The listing builds one solid part. Answer for the finished solid, in the listing's coordinates (mm). Face numbers are marked on the shaded views. A direction names the side the tool comes from. Give positions to 0.01 mm unless a question says otherwise; leave off trailing zeros. Loops run counter-clockwise (first coordinate to the right, second up) from the corner with the lowest first, then second, coordinate; pieces in that order, holes last. Notation, with made-up numbers: (51.25, 42.5) -> (90.25, 42.5) arc R19 ccw to (90.25, 48.5) -> close; hole circle Ø8 at (-37, 2). An arc over 180 degrees is marked (long way). One line per question, with ' | ' between items. Start each with the question number.
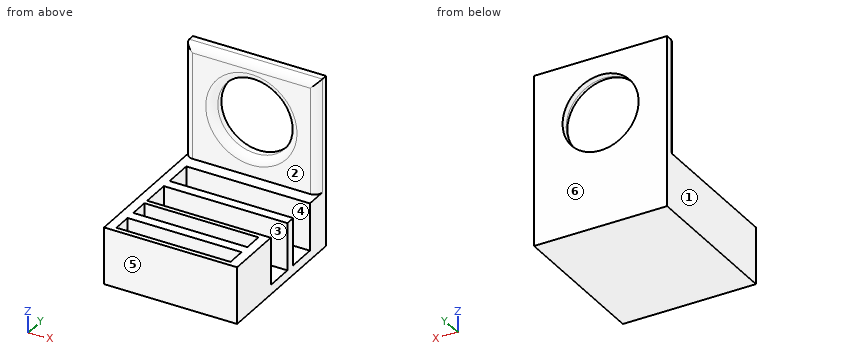
from build123d import *

# Parameters (mm, degrees)
F1_DEPTH  = 101.6
F3_DEPTH  = 31.75
F4_W      = 19.05
F4_H      = 31.75
F5_DEPTH  = 88.901
F6_W      = 88.9
F6_H      = 9.2075
F7_DEPTH  = 76.2
F8_W      = 19.05
F8_H      = 31.75
F9_DEPTH  = 6.35
F10_R     = 25.4
F11_DEPTH = 9.2085
F12_R     = 5.08


with BuildPart() as f1:
    # F0 (on Front) → F1 (new body)
    with BuildSketch(Plane.XZ):
        Polygon((44.45, 19.05), (0, 19.05), (-44.45, 19.05), (-44.45, 0), (-44.45, -19.05), (0, -19.05), (44.45, -19.05), (44.45, 0), align=None)
    extrude(amount=F1_DEPTH)

    # F2 (on face) → F3 (cut)
    with BuildSketch(Plane.XY.offset(19.05)):
        Polygon((38.1, -85.598), (0, -85.598), (-38.1, -85.598), (-38.1, -98.298), (0, -98.298), (38.1, -98.298), align=None)
        Polygon((-38.1, -78.994), (0, -78.994), (38.1, -78.994), (38.1, -66.294), (0, -66.294), (-38.1, -66.294), align=None)
    extrude(amount=-F3_DEPTH, mode=Mode.SUBTRACT)

    # F4 (on face) → F5 (cut, through all)
    with BuildSketch(Plane(origin=(-44.45, 0, 0), x_dir=(0, -1, 0), z_dir=(-1, 0, 0))):
        with Locations((53.594, 3.175)):
            Rectangle(F4_W, F4_H)
        with Locations((27.94, 3.175)):
            Rectangle(F4_W, F4_H)
    extrude(amount=-F5_DEPTH, mode=Mode.SUBTRACT)

    # F6 (on face) → F7 (join)
    with BuildSketch(Plane.XY.offset(19.05)):
        with Locations((0, -4.60375)):
            Rectangle(F6_W, F6_H)
    extrude(amount=F7_DEPTH)

    # F8 (on face) → F9 (join, through all)
    with BuildSketch(Plane(origin=(-44.45, 0, 0), x_dir=(0, -1, 0), z_dir=(-1, 0, 0))):
        with Locations((27.94, 3.175)):
            Rectangle(F8_W, F8_H)
        with Locations((53.594, 3.175)):
            Rectangle(F8_W, F8_H)
    extrude(amount=-F9_DEPTH)

    # F10 (on face) → F11 (cut, through all)
    with BuildSketch(Plane.XZ.offset(9.2075)):
        with Locations((0, 57.15)):
            Circle(F10_R)
    extrude(amount=-F11_DEPTH, mode=Mode.SUBTRACT)

    # F12
    f12_edges = [f1.edges().sort_by_distance(p)[0] for p in [
        (0, -9.2075, 95.25),
        (-44.45, -9.2075, 57.15),
        (44.45, -9.2075, 57.15),
        (-25.4, -9.2075, 57.15),
    ]]
    fillet(f12_edges, radius=F12_R)


solid = f1.part
1. The part is cut by section B-B (z = 57.15). Write down the section's boundary in (x, y).
2. Straight lines are drawn through the part: L1, parallel to Y at x = 26, z = -7 (3 decimals); L2, parallel to X at y = -2, z = 57; L3, parallel to Z at x = -39.5, y = -13.5. For each, find the intervals that lie inside material, in ascending order.
3. Each of these flat-tipped pins is pushed along its axis until it touches: pin 1 Ø6 at (x, z) = (35, 45.5) entering from +Y; pin 2 Ø15 at (x, y) = (16, -28.5) entering from +Z; pin 3 Ø14 at (x, y) = (-13, -89) entering from +Z; pin 4 Ø15 at (y, z) = (-53.5, 10.5) entering from +X. Where does it stop, or does it pass through?
4. The part is cut by section C-C (y = -29.5). Write down the section's boundary in (x, z).
5. Determine the mould class of the marked faces 4, 5 and 6 for opening direction Y: released by +Y, released by -Y, zero draft, split by the parting line, or undercut.
6. For the marked faces 1, 2 and 3, determine the directions among +Z, -Z, +X, -X, +Y, -Y from which every point of the face is accessible in a straight line to the end or side of a thin tool.
Check sheet entries:
1) outline: (-44.45, -4.13) arc R5.08 ccw to (-39.37, -9.21) -> (-30.48, -9.21) arc R5.08 ccw to (-25.4, -4.13) -> (-25.4, 0) -> (-44.45, 0) -> close; (25.4, -4.13) arc R5.08 ccw to (30.48, -9.21) -> (39.37, -9.21) arc R5.08 ccw to (44.45, -4.13) -> (44.45, 0) -> (25.4, 0) -> close
2) L1: y = -101.6 to -98.298, -85.598 to -78.994, -66.294 to -63.119, -44.069 to -37.465, -18.415 to 0 | L2: x = -44.45 to -25.4, 25.4 to 44.45 | L3: z = -19.05 to 19.05
3) pin 1: stops at y = 0 | pin 2: stops at z = -12.7 | pin 3: stops at z = 19.05 | pin 4: stops at x = -38.1
4) outline: (-44.45, -19.05) -> (44.45, -19.05) -> (44.45, -12.7) -> (-38.1, -12.7) -> (-38.1, 19.05) -> (-44.45, 19.05) -> close
5) face 4: undercut | face 5: released by -Y | face 6: released by +Y
6) face 1: +Z, -Z, -X, +Y, -Y | face 2: +Z, +X, -X, -Y | face 3: +Z, +X
